```python
from build123d import *

# Parameters (mm, degrees)
F0_R     = 22
F1_DEPTH = 8
F2_R     = 16.3
F3_DEPTH = 5
F4_R     = 2
F5_DEPTH = 25


with BuildPart() as f1:
    # F0 (on Top) → F1 (new body)
    with BuildSketch(Plane.XY):
        Circle(F0_R)
    extrude(amount=F1_DEPTH)

    # F2 (on face) → F3 (join)
    with BuildSketch(Plane.XY.offset(8)):
        Circle(F2_R)
    extrude(amount=F3_DEPTH)

    # F4 (on face) → F5 (cut)
    with BuildSketch(Plane(origin=(0, 0, 0), x_dir=(1, 0, 0), z_dir=(0, 0, -1))):
        with Locations((22, 0)):
            Circle(F4_R)
        with Locations((15.556349, -15.556349)):
            Circle(F4_R)
        with Locations((0, -22)):
            Circle(F4_R)
        with Locations((-15.556349, -15.556349)):
            Circle(F4_R)
        with Locations((-22, 0)):
            Circle(F4_R)
        with Locations((-15.556349, 15.556349)):
            Circle(F4_R)
        with Locations((0, 22)):
            Circle(F4_R)
        with Locations((15.556349, 15.556349)):
            Circle(F4_R)
    extrude(amount=-F5_DEPTH, mode=Mode.SUBTRACT)


solid = f1.part
```
CAD build for the part. Positions are in the model's coordinates, mm. A direction names the side the tool comes from. Give positions to 0.01 mm unless a question says otherwise; leave off trailing zeros. Write each loop counter-clockwise with the first axis right and the second up, starting at its lowest first coordinate (ties: lowest second). Pieces come first, ordered by that corner, then holes. Notation, with made-up numbers: M 54.25,60.25 L 65.25,60.25 A20 ccw 65.25,75.25 Z; hole C 35,26 d9. An arc over 180 degrees is marked long. Return JSON: item names as keys, results as strings. Group by question number.
(1) Flat gauge pins, fed straight in: pin 1 Ø3 at (x, z) = (-7.5, 8.5) entering from -Y; pin 2 Ø5 at (y, z) = (-13, 9.5) entering from -X. Where does each tip first touch, or does it go through?
(2) Band-saw the part on D-D (z = 10). Give the cut face in (x, y), and give its area (3 significant figures).
(3) Mould opens along X. For faces 3 (the face through (14.173, 14.112, 3.944)), 4 (the face through (0, 0, 13)), 5 (the face through (14.112, -14.173, 3.944)), 6 (the face through (20.29, -8.5, 3.94)) say: pulls with the +X half, pulls with the -X half, needs draft (parallel to the pull), parting line crosses it, or undercut.
(4) Band-saw the part on C-C (z = 6). Give the cut face in (x, y).
(5) Band-saw the part on A-A (y = 0). Give the cut face in (x, z), and give its area (3 significant figures).
(6) 3-axis set-ups, long thin cutter, end or side, ignore diameter. For faces 1 (the face through (8.33, -20.36, 3.94)), 2 (the face through (-12.935, -9.918, 10.465)): which of +Z, -Z, +X, -X, +Y, -Y reach the whole face in a straight line?
(7) Drill centre lines: L1, parallel to Z at x = -13.5, y = 14; L2, parallel to Y at x = 7, z = 6.5; L3, parallel to X at y = 5, z = 4.25. Where is each one in solid material? Low to high. Write a range as [from, to].
Entries:
{
 "1": {"pin 1": "stops at y = -21.14", "pin 2": "stops at x = -19.05"},
 "2": {"outline": "C 0,0 d32.6", "area": "835 mm^2"},
 "3": {"face 3": "undercut", "face 4": "needs draft", "face 5": "undercut", "face 6": "pulls with the +X half"},
 "4": {"outline": "M -21.91,-2 A22 ccw -16.9,-14.08 A2 cw -14.08,-16.9 A22 ccw -2,-21.91 A2 cw 2,-21.91 A22 ccw 14.08,-16.9 A2 cw 16.9,-14.08 A22 ccw 21.91,-2 A2 cw 21.91,2 A22 ccw 16.9,14.08 A2 cw 14.08,16.9 A22 ccw 2,21.91 A2 cw -2,21.91 A22 ccw -14.08,16.9 A2 cw -16.9,14.08 A22 ccw -21.91,2 A2 cw Z"},
 "5": {"outline": "M -20,0 L 20,0 L 20,8 L 16.3,8 L 16.3,13 L -16.3,13 L -16.3,8 L -20,8 Z", "area": "483 mm^2"},
 "6": {"face 1": "+Z, -Z, +X, -Y", "face 2": "+Z"},
 "7": {"L1": "z = [0, 8]", "L2": "y = [-20.86, 20.86]", "L3": "x = [-21.42, 21.42]"}
}
